Model file for the job. Use its own axes, mm. Give positions to 0.01 mm unless a question says otherwise; leave off trailing zeros. Loops run counter-clockwise (first coordinate to the right, second up) from the corner with the lowest first, then second, coordinate; pieces in that order, holes last. Notation, with made-up numbers: (-27, 26) -> (-1, 26) arc R23 ccw to (-1, 50) -> close; hole circle Ø2 at (-27.75, 41). An arc over 180 degrees is marked (long way). Use CSV: the item, a comma, the result in double quotes. Start each with the question number.
(1) Cut at A-A on x = -20.75. Write the cut outline in (y, z), then the cut area to 3 significant figures.
(2) Cut at B-B on y = 4. Write the cut outline in (x, z).
(3) Drill centre lines: probe 1 along Z at (x, y) = (-22.25, 4.5); probe 2 along Y at (x, z) = (-27.75, 0.1); probe 3 along Y at (x, z) = (-20.75, 0.15). Where is each one in solid material? Low to high.
(4) Cut at C-C on z = 0.15. Write the cut outline in (x, y).
from build123d import *

# Parameters (mm, degrees)
SKETCH1_R           = 4.88
BOSS_EXTRUDE1_DEPTH = 0.2
BOSS_EXTRUDE2_DEPTH = 0.001


with BuildPart() as part:
    # Sketch1 → Boss-Extrude1 (new body)
    with BuildSketch(Plane.XY):
        with Locations((-23.609402801, 8.006667037)):
            Circle(SKETCH1_R)
    extrude(amount=BOSS_EXTRUDE1_DEPTH)

    # Sketch2 → Boss-Extrude2 (add)
    with BuildSketch(Plane.XY.offset(0.2)):
        with BuildLine():
            Line((-24.638921092, 9.949558898), (-23.847354586, 9.949558898))
            add(Edge.make_bspline(
                [(-23.847354586, 9.949558898), (-23.785642872, 9.949127512), (-23.666353431, 9.948293638), (-23.493526632, 9.938897884), (-23.3328197, 9.92444788), (-23.184129043, 9.904569281), (-23.047759499, 9.878264451), (-22.923886914, 9.845270197), (-22.812095543, 9.80718382), (-22.711159616, 9.762367469), (-22.619014823, 9.710116054), (-22.531520401, 9.651912174), (-22.448848143, 9.585623648), (-22.369837876, 9.512529316), (-22.295509243, 9.431291939), (-22.224624407, 9.343257102), (-22.158918949, 9.247148179), (-22.096406736, 9.145269558), (-22.039872757, 9.037189487), (-21.990561709, 8.923827923), (-21.949253545, 8.805914387), (-21.915688522, 8.683323216), (-21.888933325, 8.556461375), (-21.870213253, 8.425072869), (-21.858640318, 8.28927934), (-21.857466341, 8.197245399), (-21.85686981, 8.150480373)],
                knots=[0, 0, 0, 0, 1.44355588, 2.790409838, 4.047694926, 5.217575253, 6.298404546, 7.294384826, 8.214239204, 9.058592145, 9.873746385, 10.689560431, 11.514393297, 12.350027578, 13.205127629, 14.088021785, 14.991911688, 15.926770944, 16.882954281, 17.842803888, 18.816321264, 19.80318086, 20.814351908, 21.847355356, 22.906180909, 24, 24, 24, 24], degree=3))
            add(Edge.make_bspline(
                [(-21.85686981, 8.150480373), (-21.85843185, 8.084491877), (-21.861506817, 7.954589661), (-21.88740862, 7.763959656), (-21.929300607, 7.581221782), (-21.988204545, 7.407805488), (-22.06122966, 7.245255069), (-22.148466338, 7.096437035), (-22.248635484, 6.962150166), (-22.360570124, 6.8430631), (-22.481768076, 6.740706152), (-22.607717189, 6.653044917), (-22.739644436, 6.583916719), (-22.855890777, 6.540079104), (-22.956690858, 6.5128159), (-23.045192238, 6.496703084), (-23.145720776, 6.481926659), (-23.259213813, 6.470507757), (-23.38517348, 6.460324902), (-23.524101853, 6.454791935), (-23.675549121, 6.45019486), (-23.780743569, 6.44977644), (-23.835435515, 6.449558898)],
                knots=[0, 0, 0, 0, 1.315458931, 2.589557908, 3.828601765, 5.048913369, 6.235739168, 7.376350998, 8.481830359, 9.569842114, 10.627874879, 11.640079404, 12.624025415, 13.590060155, 14.111227486, 14.704434459, 15.382649715, 16.137166398, 16.978595427, 17.902333227, 18.909396075, 20, 20, 20, 20], degree=3))
            Line((-23.835435515, 6.449558898), (-24.638921092, 6.449558898))
            Line((-24.638921092, 6.449558898), (-24.638921092, 9.949558898))
        make_face()
        with BuildLine():
            Line((-24.010715964, 9.32135377), (-24.010715964, 7.077764027))
            Line((-24.010715964, 7.077764027), (-23.682590964, 7.077764027))
            add(Edge.make_bspline(
                [(-23.682590964, 7.077764027), (-23.643549128, 7.077835567), (-23.568458681, 7.077973164), (-23.460045072, 7.084527018), (-23.359789974, 7.09110528), (-23.267969364, 7.103591041), (-23.183915, 7.1174993), (-23.10878157, 7.136854547), (-23.041020248, 7.157185594), (-22.981458724, 7.183069538), (-22.92690522, 7.212203639), (-22.876394908, 7.246337615), (-22.827638314, 7.284242109), (-22.781546984, 7.327031945), (-22.737946472, 7.374140505), (-22.697094746, 7.425810519), (-22.658446545, 7.48188434), (-22.622993894, 7.542658445), (-22.590597072, 7.607491044), (-22.56185746, 7.675754141), (-22.538028081, 7.748016219), (-22.518222561, 7.823600818), (-22.50406927, 7.903165988), (-22.492360122, 7.986122401), (-22.486323715, 8.072798724), (-22.485495256, 8.131776191), (-22.485074938, 8.161698321)],
                knots=[0, 0, 0, 0, 1.50275155, 2.890291501, 4.180787663, 5.369391935, 6.45668281, 7.458360028, 8.354766181, 9.177074746, 9.954075863, 10.732690366, 11.5210699, 12.329727389, 13.151100085, 13.990027547, 14.863562427, 15.770965086, 16.696477834, 17.652329173, 18.619756807, 19.62365428, 20.657822005, 21.729286259, 22.847956731, 24, 24, 24, 24], degree=3))
            add(Edge.make_bspline(
                [(-22.485074938, 8.161698321), (-22.485912068, 8.207551158), (-22.487544407, 8.296960637), (-22.503286326, 8.427187495), (-22.528911167, 8.54981559), (-22.565475347, 8.664389817), (-22.611565628, 8.77123219), (-22.66925836, 8.869437527), (-22.736070668, 8.960655544), (-22.788904019, 9.014166959), (-22.815303304, 9.040905052)],
                knots=[0, 0, 0, 0, 1.13821349, 2.219428113, 3.251817212, 4.244760574, 5.201143372, 6.134805572, 7.068016741, 8, 8, 8, 8], degree=3))
            add(Edge.make_bspline(
                [(-22.815303304, 9.040905052), (-22.841335498, 9.063689523), (-22.894503307, 9.110224223), (-22.987848507, 9.165984695), (-23.090710084, 9.214975736), (-23.205441201, 9.253820167), (-23.330933033, 9.284539999), (-23.467933013, 9.305726716), (-23.615707474, 9.319341076), (-23.718082178, 9.320668499), (-23.77093231, 9.32135377)],
                knots=[0, 0, 0, 0, 0.813307809, 1.661089106, 2.549956539, 3.493439533, 4.508053171, 5.589449661, 6.755572447, 8, 8, 8, 8], degree=3))
            Line((-23.77093231, 9.32135377), (-24.010715964, 9.32135377))
        make_face(mode=Mode.SUBTRACT)
    extrude(amount=BOSS_EXTRUDE2_DEPTH)


solid = part.part
Check result:
1,outline,"(4.05, 0) -> (11.96, 0) -> (11.96, 0.2) -> (4.05, 0.2) -> close"
1,area,"1.58 mm²"
2,outline,"(-26.4, 0) -> (-20.82, 0) -> (-20.82, 0.2) -> (-26.4, 0.2) -> close"
3,probe 1,"0 to 0.2"
3,probe 2,"5.42 to 10.59"
3,probe 3,"4.05 to 11.96"
4,outline,"circle Ø9.76 at (-23.61, 8.01)"
